from build123d import *

# Parameters (mm, degrees)
SKETCH1_R           = 2.1
BOSS_EXTRUDE1_DEPTH = 6.35
SKETCH2_R           = 1.6
CUT_EXTRUDE1_DEPTH  = 65.6
SKETCH3_R           = 3
CUT_EXTRUDE2_DEPTH  = 2.5
SKETCH4_R           = 1.5
CUT_EXTRUDE3_DEPTH  = 5
FILLET1_R           = 1


with BuildPart() as part:
    # Sketch1 → Boss-Extrude1 (new body)
    with BuildSketch(Plane.XY):
        with BuildLine():
            Line((45.4, -16), (45.4, -29))
            Line((45.4, -29), (110, -29))
            Line((110, -29), (110, -1))
            Line((110, -1), (104, -1))
            Line((104, -1), (104, -2.645898034))
            ThreePointArc((104, -2.645898034), (106.5, -6), (104, -9.354101966))
            Line((104, -9.354101966), (104, -16))
            Line((104, -16), (99, -16))
            Line((99, -16), (45.4, -16))
        make_face()
        with Locations((96.978626472, -22.5)):
            Circle(SKETCH1_R, mode=Mode.SUBTRACT)
        with Locations((83.957252945, -22.5)):
            Circle(SKETCH1_R, mode=Mode.SUBTRACT)
        with Locations((70.935879417, -22.5)):
            Circle(SKETCH1_R, mode=Mode.SUBTRACT)
    extrude(amount=BOSS_EXTRUDE1_DEPTH)

    # Sketch2 → Cut-Extrude1 (cut, through all)
    with BuildSketch(Plane(origin=(110, 0, 0), x_dir=(0, 0, -1), z_dir=(1, 0, 0))):
        with Locations((-3.175, -12)):
            Circle(SKETCH2_R)
    extrude(amount=-CUT_EXTRUDE1_DEPTH, mode=Mode.SUBTRACT)

    # Sketch3 → Cut-Extrude2 (cut)
    with BuildSketch(Plane(origin=(110, 0, 0), x_dir=(0, 0, -1), z_dir=(1, 0, 0))):
        with Locations((-3.175, -12)):
            Circle(SKETCH3_R)
    extrude(amount=-CUT_EXTRUDE2_DEPTH, mode=Mode.SUBTRACT)

    # Sketch4 → Cut-Extrude3 (cut)
    with BuildSketch(Plane(origin=(110, 0, 0), x_dir=(0, 0, -1), z_dir=(1, 0, 0))):
        with Locations((-3.175, -17.5)):
            Circle(SKETCH4_R)
        with Locations((-3.175, -6.5)):
            Circle(SKETCH4_R)
    extrude(amount=-CUT_EXTRUDE3_DEPTH, mode=Mode.SUBTRACT)

    # Fillet1
    fillet1_edges = [part.edges().sort_by_distance(p)[0] for p in [
        (104, -9.354101966, 3.175),
        (104, -2.645898034, 3.175),
    ]]
    fillet(fillet1_edges, radius=FILLET1_R)


solid = part.part
Can you work these out from the model? Positions are in its coordinate system, mm. A direction names the side the tool comes from. Round coordinates to 2 decimals unless told otherwise and drop trailing zeros. Order: outer loops, then holes, each group sorted by start corner. A loop starts at its lowest first (then second) coordinate and runs counter-clockwise, first axis right, second up. Notation, with made-up numbers: (70, 26) -> (90, 26) arc R28 cw to (90, 50) -> close; hole circle Ø11 at (19, 82). An arc over 180 degrees is marked (long way). Write each question's results on one line, items separated by ' | '. Start each with the question number.
Item 1: If we section it at A-A, the plane y = -22.5: Write out the boundary of the cut face in (x, z), then the cut area to 3 significant figures.
Item 2: Which directions (+Z, -Z, +X, -X, +Y, -Y) give clear straight access to the entire face, cutting with the end or side of a thin tool? Please do faces 1 (the flat face through (104, -14, 3)), 2 (the cylindrical face through (106.056, -4.294, 3.131)), 3 (the flat face through (105, -17, 3)).
Item 3: If we section it at D-D, the plane y = -12: Write out the boundary of the cut face in (x, z) (3 decimals), then the cut area to 3 significant figures.
Item 4: Will these pins go through, and if not, where does the flat tip stop? pin 1 (1.5 mm diameter, centred on y = -18, z = 4, fed in from +X); pin 2 (3 mm diameter, centred on y = -6, z = 2, fed in from -X); pin 3 (0.8 mm diameter, centred on y = -1.5, z = 2, fed in from -X).
Item 5: Thinking about a two-plate mould opening in Y: for faces 4 (the flat face through (77, -29, 3)), 5 (the cylindrical face through (108.768, -11.099, 0.314)), 6 (the flat face through (107.5, -13.3, 1.9)), 7 (the flat face through (110, -15.2, 3.1)), which applies, +Y half, -Y half, draft (parallel to the pull), parting line (faces both ways), or undercut?
Item 6: If we section it at B-B, the plane z = 2.75: State how many separate pieces and enclosed holes the cut face has, then the cut area to 3 significant figures.
Item 7: Please list where these lines run through material, in increasing order: L1, parallel to Y at x = 97, z = 0.5; L2, parallel to X at y = -20.75, z = 5; L3, parallel to X at y = -21.75, z = 5.5.
Item 8: If we section it at C-C, the plane x = 85: Write out the boundary of the cut face in (y, z), then the cut area to 3 significant figures.
Results:
1) outline: (45.4, 0) -> (68.84, 0) -> (68.84, 6.35) -> (45.4, 6.35) -> close; (73.04, 0) -> (81.86, 0) -> (81.86, 6.35) -> (73.04, 6.35) -> close; (86.06, 0) -> (94.88, 0) -> (94.88, 6.35) -> (86.06, 6.35) -> close; (99.08, 0) -> (110, 0) -> (110, 6.35) -> (99.08, 6.35) -> close | area: 330 mm2
2) face 1: +Z, -Z, -X, +Y | face 2: +Z, -Z, -X | face 3: +X
3) outline: (104, 0) -> (110, 0) -> (110, 0.175) -> (107.5, 0.175) -> (107.5, 1.575) -> (104, 1.575) -> close; (104, 4.775) -> (107.5, 4.775) -> (107.5, 6.175) -> (110, 6.175) -> (110, 6.35) -> (104, 6.35) -> close | area: 11.9 mm2
4) pin 1: stops at x = 110 | pin 2: stops at x = 106.16 | pin 3: stops at x = 104
5) face 4: -Y half | face 5: undercut | face 6: undercut | face 7: draft
6) separate pieces: 3 | enclosed holes: 3 | area: 825 mm2
7) L1: y = -29 to -24.6, -20.4 to -16 | L2: x = 45.4 to 69.78, 72.1 to 82.8, 85.12 to 95.82, 98.14 to 110 | L3: x = 45.4 to 68.97, 72.9 to 82, 85.92 to 95.02, 98.94 to 110
8) outline: (-29, 0) -> (-24.32, 0) -> (-24.32, 6.35) -> (-29, 6.35) -> close; (-20.68, 0) -> (-16, 0) -> (-16, 6.35) -> (-20.68, 6.35) -> close | area: 59.4 mm2
